For this review, take the finished solid that the model builds, in its own axes (mm). Face numbers are marked on the shaded views. A direction names the side the tool comes from. Coordinates: 2 decimals unless noted, no trailing zeros. Loops run counter-clockwise (first coordinate to the right, second up) from the corner with the lowest first, then second, coordinate; pieces in that order, holes last. Notation, with made-up numbers: (5, 22.5) - (45, 22.5) arc R20 cw to (45, 36.5) - close; hole circle Ø4 at (78, -5). An arc over 180 degrees is marked (long way). One line per item, written item: value. Start each with the question number.
1. Insertion check: pin 1 (4 mm diameter, centred on x = -11.5, y = 25.5, fed in from +Z); pin 2 (4 mm diameter, centred on x = -12, z = -3.5, fed in from +Y); pin 3 (3 mm diameter, centred on y = 7.5, z = 2.5, fed in from -X). Each pin has a flat end and moves straight along its axis. Give the tip position at first contact, or say it passes through.
2. Take a section at A-A, the plane x = 78.5. State the section outline as (y, z) points.
3. Take a section at B-B, the plane y = 26.5. State the section outline as (x, z) points.
4. The part is to be moulded in two halves that separate along X. For the marked faces 1 and 2, say which applies: released by +X, released by -X, zero draft, split by the parting line, or undercut.
5. For the marked faces 3 and 4, list the 3-axis set-ups (+Z, -Z, +X, -X, +Y, -Y) from which the entire face can be reached by the end or side of a thin tool; tool diameter is ignored.
6. To check wall thickness, follow line 1 (X direction, y = 30, z = -56.5); line 2 (Y direction, x = 78.5, z = -60.85); line 3 (Y direction, x = 51, z = -30). State the ranges of each line that lie inside material, in increasing order. Write a range as from..to.
7. Take a section at D-D, the plane x = 14. State the section outline as (y, z) points.
8. Take a section at C-C, the plane z = -14. State the section outline as (x, y) points, and give its area (3 significant figures).
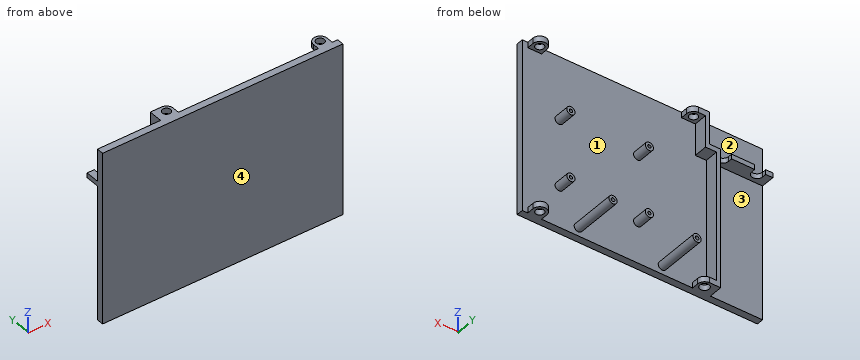
```python
from build123d import *

# Parameters (mm, degrees)
SKETCH1_W           = 175
SKETCH1_H           = 125
BOSS_EXTRUDE1_DEPTH = 5
BOSS_EXTRUDE2_DEPTH = 10
SKETCH3_R           = 3.41
SKETCH3_R_2         = 3
BOSS_EXTRUDE3_DEPTH = 4
BOSS_EXTRUDE4_START = -4
SKETCH4_R           = 3
BOSS_EXTRUDE4_DEPTH = 4
SKETCH5_R           = 3
SKETCH5_R_2         = 1.2
BOSS_EXTRUDE5_DEPTH = 11.4
SKETCH6_R           = 3
SKETCH6_R_2         = 1.35
BOSS_EXTRUDE6_DEPTH = 33.7
CUT_EXTRUDE1_REACH  = 138.96


with BuildPart() as part:
    # Sketch1 → Boss-Extrude1 (new body)
    with BuildSketch(Plane(origin=(0, 0, 0), x_dir=(1, 0, 0), z_dir=(0, 1, 0))):
        Rectangle(SKETCH1_W, SKETCH1_H)
    extrude(amount=BOSS_EXTRUDE1_DEPTH)

    # Sketch2 → Boss-Extrude2 (add)
    with BuildSketch(Plane(origin=(0, 5, 0), x_dir=(1, 0, 0), z_dir=(0, 1, 0))):
        Polygon((-49.5, 62.5), (-49.5, -35.5), (-87.5, -35.5), (-87.5, -39), (-41.5, -39), (-41.5, -62.5), (-38.5, -62.5), (-38.5, -35.5), (-46.5, -35.5), (-46.5, 62.5), align=None)
    extrude(amount=BOSS_EXTRUDE2_DEPTH)

    # Sketch3 → Boss-Extrude3 (add)
    # profile 1 of 2: a face of its own
    with BuildSketch(Plane(origin=(0, 0, -62.5), x_dir=(-1, 0, 0), z_dir=(0, 0, -1))):
        with BuildLine():
            Line((46.5, 5), (36.5, 5))
            Line((36.5, 5), (36.5, 10))
            ThreePointArc((36.5, 10), (37.964466094, 13.535533906), (41.5, 15))
            Line((41.5, 15), (46.5, 15))
            Line((46.5, 15), (46.5, 5))
        make_face()
        with Locations((41.5, 10)):
            Circle(SKETCH3_R, mode=Mode.SUBTRACT)
    # profile 2 of 2: a face of its own
    with BuildSketch(Plane(origin=(0, 0, -62.5), x_dir=(-1, 0, 0), z_dir=(0, 0, -1))):
        with BuildLine():
            Line((-83.5, 10), (-83.5, 5))
            Line((-83.5, 5), (-73.5, 5))
            Line((-73.5, 5), (-73.5, 10))
            ThreePointArc((-73.5, 10), (-78.5, 15), (-83.5, 10))
        make_face()
        with Locations(Location((-78.5, 10, 0), (0, 0, 180))):
            Circle(SKETCH3_R_2, mode=Mode.SUBTRACT)
    extrude(amount=-BOSS_EXTRUDE3_DEPTH)

    # Sketch4 → Boss-Extrude4 (add)
    # profile 1 of 2: a face of its own
    with BuildSketch(Plane.XY.offset(62.5).offset(BOSS_EXTRUDE4_START)):
        with BuildLine():
            Line((73.5, 5), (83.5, 5))
            Line((83.5, 5), (83.5, 10))
            ThreePointArc((83.5, 10), (78.5, 15), (73.5, 10))
            Line((73.5, 10), (73.5, 5))
        make_face()
        with Locations((78.5, 10)):
            Circle(SKETCH4_R, mode=Mode.SUBTRACT)
    # profile 2 of 2: a face of its own
    with BuildSketch(Plane.XY.offset(62.5).offset(BOSS_EXTRUDE4_START)):
        with BuildLine():
            Line((-38.5, 15), (-38.5, 5))
            Line((-38.5, 5), (-28.5, 5))
            Line((-28.5, 5), (-28.5, 10))
            ThreePointArc((-28.5, 10), (-29.964466094, 13.535533906), (-33.5, 15))
            Line((-33.5, 15), (-38.5, 15))
        make_face()
        with Locations((-33.5, 10)):
            Circle(SKETCH4_R, mode=Mode.SUBTRACT)
    extrude(amount=BOSS_EXTRUDE4_DEPTH)

    # Sketch5 → Boss-Extrude5 (add)
    # profile 1 of 4: a face of its own
    with BuildSketch(Plane(origin=(0, 5, 0), x_dir=(1, 0, 0), z_dir=(0, 1, 0))):
        with Locations(Location((3.5, 32.9, 0), (0, 0, 90))):
            Circle(SKETCH5_R)
        with Locations(Location((3.5, 32.9, 0), (0, 0, 90))):
            Circle(SKETCH5_R_2, mode=Mode.SUBTRACT)
    # profile 2 of 4: a face of its own
    with BuildSketch(Plane(origin=(0, 5, 0), x_dir=(1, 0, 0), z_dir=(0, 1, 0))):
        with Locations(Location((60.65, 32.9, 0), (0, 0, 90))):
            Circle(SKETCH5_R)
        with Locations(Location((60.65, 32.9, 0), (0, 0, 90))):
            Circle(SKETCH5_R_2, mode=Mode.SUBTRACT)
    # profile 3 of 4: a face of its own
    with BuildSketch(Plane(origin=(0, 5, 0), x_dir=(1, 0, 0), z_dir=(0, 1, 0))):
        with Locations(Location((60.65, -15.868, 0), (0, 0, 90))):
            Circle(SKETCH5_R)
        with Locations(Location((60.65, -15.868, 0), (0, 0, 90))):
            Circle(SKETCH5_R_2, mode=Mode.SUBTRACT)
    # profile 4 of 4: a face of its own
    with BuildSketch(Plane(origin=(0, 5, 0), x_dir=(1, 0, 0), z_dir=(0, 1, 0))):
        with Locations(Location((3.5, -15.868, 0), (0, 0, 90))):
            Circle(SKETCH5_R)
        with Locations(Location((3.5, -15.868, 0), (0, 0, 90))):
            Circle(SKETCH5_R_2, mode=Mode.SUBTRACT)
    extrude(amount=BOSS_EXTRUDE5_DEPTH)

    # Sketch6 → Boss-Extrude6 (add)
    # profile 1 of 2: a face of its own
    with BuildSketch(Plane(origin=(0, 5, 0), x_dir=(1, 0, 0), z_dir=(0, 1, 0))):
        with Locations(Location((46.7, 56.5, 0), (0, 0, 270))):
            Circle(SKETCH6_R)
        with Locations(Location((46.7, 56.5, 0), (0, 0, 270))):
            Circle(SKETCH6_R_2, mode=Mode.SUBTRACT)
    # profile 2 of 2: a face of its own
    with BuildSketch(Plane(origin=(0, 5, 0), x_dir=(1, 0, 0), z_dir=(0, 1, 0))):
        with Locations(Location((-14.5, 56.5, 0), (0, 0, 270))):
            Circle(SKETCH6_R)
        with Locations(Location((-14.5, 56.5, 0), (0, 0, 270))):
            Circle(SKETCH6_R_2, mode=Mode.SUBTRACT)
    extrude(amount=BOSS_EXTRUDE6_DEPTH)

    # Sketch7 → Cut-Extrude1 (cut, up to next)
    with BuildSketch(Plane(origin=(0, 0, 35.5), x_dir=(-1, 0, 0), z_dir=(0, 0, -1)), mode=Mode.PRIVATE) as cut_extrude1_sk1:
        with BuildLine():
            Line((49.5, 15), (49.5, 12))
            ThreePointArc((49.5, 12), (53.5, 8), (57.5, 12))
            Line((57.5, 12), (57.5, 15))
            Line((57.5, 15), (49.5, 15))
        make_face()
    cut_extrude1_tool1 = extrude(cut_extrude1_sk1.sketch, amount=-CUT_EXTRUDE1_REACH, mode=Mode.PRIVATE) & part.part
    # Sketch7 → Cut-Extrude1 (cut, up to next)
    with BuildSketch(Plane(origin=(0, 0, 35.5), x_dir=(-1, 0, 0), z_dir=(0, 0, -1)), mode=Mode.PRIVATE) as cut_extrude1_sk2:
        with BuildLine():
            Line((74.3, 15), (74.3, 12))
            ThreePointArc((74.3, 12), (78.3, 8), (82.3, 12))
            Line((82.3, 12), (82.3, 15))
            Line((82.3, 15), (74.3, 15))
        make_face()
    cut_extrude1_tool2 = extrude(cut_extrude1_sk2.sketch, amount=-CUT_EXTRUDE1_REACH, mode=Mode.PRIVATE) & part.part
    add(cut_extrude1_tool1.solids().sort_by_distance((-53.5, 11.864313, 35.5))[0], mode=Mode.SUBTRACT)
    add(cut_extrude1_tool2.solids().sort_by_distance((-78.3, 11.864313, 35.5))[0], mode=Mode.SUBTRACT)


solid = part.part
```
Solutions:
1. pin 1: z = -53.67
1. pin 2: y = 5
1. pin 3: x = -49.5
2. outline: (0, -62.5) - (7, -62.5) - (7, -58.5) - (5, -58.5) - (5, 58.5) - (7, 58.5) - (7, 62.5) - (0, 62.5) - close; (13, -62.5) - (15, -62.5) - (15, -58.5) - (13, -58.5) - close; (13, 58.5) - (15, 58.5) - (15, 62.5) - (13, 62.5) - close
3. outline: circle Ø6 at (-14.5, -56.5); circle Ø6 at (46.7, -56.5); hole circle Ø2.7 at (-14.5, -56.5); hole circle Ø2.7 at (46.7, -56.5)
4. face 1: undercut
4. face 2: zero draft
5. face 3: -Z, -X, +Y
5. face 4: +Z, -Z, +X, -X, -Y
6. line 1: -17.5..-15.85, -13.15..-11.5, 43.7..45.35, 48.05..49.7
6. line 2: 0..7, 13..15
6. line 3: 0..5
7. outline: (0, -62.5) - (5, -62.5) - (5, 62.5) - (0, 62.5) - close
8. outline: (-87.5, 0) - (87.5, 0) - (87.5, 5) - (-46.5, 5) - (-46.5, 15) - (-49.5, 15) - (-49.5, 5) - (-87.5, 5) - close
8. area: 905 mm2
